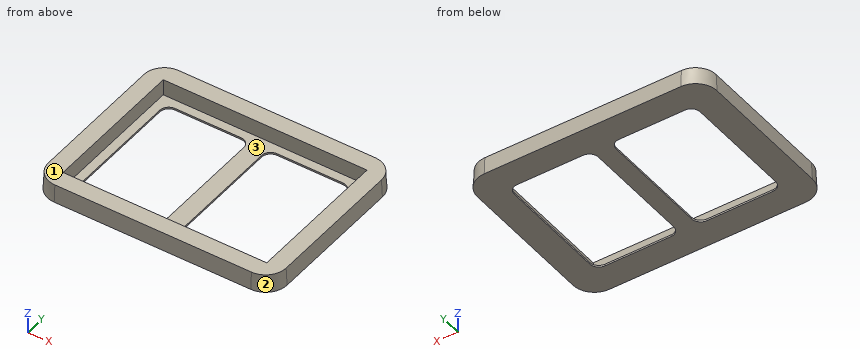
from build123d import *

# Parameters (mm, degrees)
F1_DEPTH = 10
F1_TAPER = 3
F2_W     = 114
F2_H     = 81
F3_DEPTH = 9
F5_DEPTH = 1


with BuildPart() as f1:
    # F0 (on Top) → F1 (new body)
    with BuildSketch(Plane.XY):
        with BuildLine():
            Line((55, 50.5), (-55, 50.5))
            ThreePointArc((-55, 50.5), (-63.4852813742, 46.9852813742), (-67, 38.5))
            Line((-67, 38.5), (-67, -38.5))
            ThreePointArc((-67, -38.5), (-63.4852813742, -46.9852813742), (-55, -50.5))
            Line((-55, -50.5), (55, -50.5))
            ThreePointArc((55, -50.5), (63.4852813742, -46.9852813742), (67, -38.5))
            Line((67, -38.5), (67, 38.5))
            ThreePointArc((67, 38.5), (63.4852813742, 46.9852813742), (55, 50.5))
        make_face()
    extrude(amount=F1_DEPTH, taper=F1_TAPER)

    # F2 (on face) → F3 (cut)
    with BuildSketch(Plane.XY.offset(10)):
        Rectangle(F2_W, F2_H)
    extrude(amount=-F3_DEPTH, mode=Mode.SUBTRACT)

    # F4 (on face) → F5 (cut, through all)
    with BuildSketch(Plane.XY.offset(1)):
        with BuildLine():
            ThreePointArc((52, 30.5), (50.5355339059, 34.0355339059), (47, 35.5))
            Line((47, 35.5), (10, 35.5))
            ThreePointArc((10, 35.5), (6.4644660941, 34.0355339059), (5, 30.5))
            Line((5, 30.5), (5, -30.5))
            ThreePointArc((5, -30.5), (6.4644660941, -34.0355339059), (10, -35.5))
            Line((10, -35.5), (47, -35.5))
            ThreePointArc((47, -35.5), (50.5355339059, -34.0355339059), (52, -30.5))
            Line((52, -30.5), (52, 30.5))
        make_face()
        with BuildLine():
            Line((-5, -30.5), (-5, 30.5))
            ThreePointArc((-5, 30.5), (-6.4644660941, 34.0355339059), (-10, 35.5))
            Line((-10, 35.5), (-47, 35.5))
            ThreePointArc((-47, 35.5), (-50.5355339059, 34.0355339059), (-52, 30.5))
            Line((-52, 30.5), (-52, -30.5))
            ThreePointArc((-52, -30.5), (-50.5355339059, -34.0355339059), (-47, -35.5))
            Line((-47, -35.5), (-10, -35.5))
            ThreePointArc((-10, -35.5), (-6.4644660941, -34.0355339059), (-5, -30.5))
        make_face()
    extrude(amount=-F5_DEPTH, mode=Mode.SUBTRACT)


solid = f1.part
Verification items for the finished model (mm, model axes). Face numbers are marked on the shaded views. Give positions to 0.01 mm unless a question says otherwise; leave off trailing zeros. Write each loop counter-clockwise with the first axis right and the second up, starting at its lowest first coordinate (ties: lowest second). Pieces come first, ordered by that corner, then holes.
(1) Gauge pin test, flat ends, axial feed: pin 1 (0.8 mm diameter, centred on x = 21, z = 0.5, fed in from +Y); pin 2 (4.5 mm diameter, centred on x = 18.5, z = 5.5, fed in from -Y); pin 3 (0.8 mm diameter, centred on y = -3.5, z = 0.5, fed in from -X). Record the tip position at first contact, or that the pin passes through.
(2) Material ranges on line 1 (X direction, y = -29.5, z = 0.5); line 2 (Y direction, x = -56, z = 9.25); line 3 (X direction, y = -5.5, z = 5.25), recorded low to high.
(3) Cross-section at D-D (x = 49). Enter the section's corners in (y, z), plus the area to 3 significant figures.
(4) Cross-section at A-A (x = -13.5). Enter the section's corners in (y, z).
(5) Cross-section at B-B (y = -2). Enter the section's corners in (x, z), plus the area to 3 significant figures.
(6) Cross-section at C-C (z = 4). Enter the section's corners in (x, y).
(7) Mould release check, pull along X, two halves, no side actions. Record for the marked faces 1, 2 and 3: +X half, -X half, draft (parallel to the pull), parting line (faces both ways), or undercut.
Worked out:
1. pin 1: stops at y = 50.49
1. pin 2: stops at y = -50.33
1. pin 3: stops at x = -66.99
2. line 1: x = -66.97 to -52, -5 to 5, 52 to 66.97
2. line 2: y = -49.97 to -40.5, 40.5 to 49.97
2. line 3: x = -66.72 to -57, 57 to 66.72
3. outline: (-50.5, 0) - (-35.08, 0) - (-35.08, 1) - (-40.5, 1) - (-40.5, 10) - (-49.98, 10) - close; (35.08, 0) - (50.5, 0) - (49.98, 10) - (40.5, 10) - (40.5, 1) - (35.08, 1) - close
3. area: 206 mm2
4. outline: (-50.5, 0) - (-35.5, 0) - (-35.5, 1) - (-40.5, 1) - (-40.5, 10) - (-49.98, 10) - close; (35.5, 0) - (50.5, 0) - (49.98, 10) - (40.5, 10) - (40.5, 1) - (35.5, 1) - close
5. outline: (-67, 0) - (-52, 0) - (-52, 1) - (-57, 1) - (-57, 10) - (-66.48, 10) - close; (-5, 0) - (5, 0) - (5, 1) - (-5, 1) - close; (52, 0) - (67, 0) - (66.48, 10) - (57, 10) - (57, 1) - (52, 1) - close
5. area: 215 mm2
6. outline: (-66.79, -38.5) arc R11.79 ccw to (-55, -50.29) - (55, -50.29) arc R11.79 ccw to (66.79, -38.5) - (66.79, 38.5) arc R11.79 ccw to (55, 50.29) - (-55, 50.29) arc R11.79 ccw to (-66.79, 38.5) - close; hole (-57, -40.5) - (57, -40.5) - (57, 40.5) - (-57, 40.5) - close
7. face 1: draft
7. face 2: +X half
7. face 3: undercut
